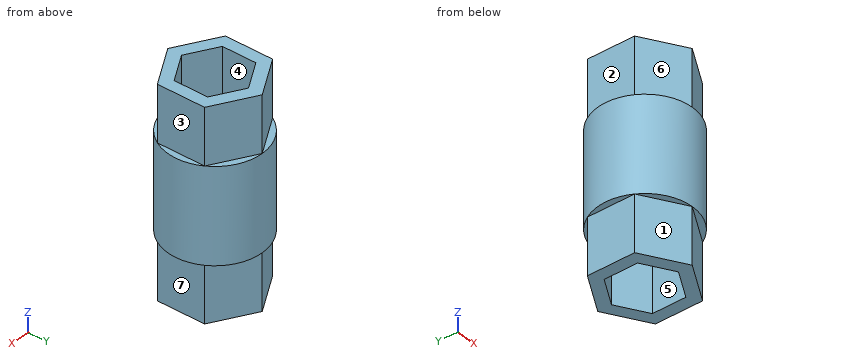
```python
from build123d import *

# Parameters (mm, degrees)
SKETCH1_R           = 11
SKETCH1_R_2         = 6.4
BOSS_EXTRUDE1_DEPTH = 11
BOSS_EXTRUDE2_DEPTH = 24
CUT_EXTRUDE3_DEPTH  = 49


with BuildPart() as part:
    # Sketch1 → Boss-Extrude1 (new body, symmetric)
    with BuildSketch(Plane.XY):
        Circle(SKETCH1_R)
        Circle(SKETCH1_R_2, mode=Mode.SUBTRACT)
    extrude(amount=BOSS_EXTRUDE1_DEPTH, both=True)

    # Sketch1_3 → Boss-Extrude2 (add, symmetric)
    with BuildSketch(Plane.XY):
        Polygon((0, -11), (9.526279442, -5.5), (9.526279442, 5.5), (0, 11), (-9.526279442, 5.5), (-9.526279442, -5.5), align=None)
    extrude(amount=BOSS_EXTRUDE2_DEPTH, both=True)

    # Sketch2 → Cut-Extrude3 (cut, through all)
    with BuildSketch(Plane.XY.offset(24)):
        Polygon((0, -7.8), (6.75499815, -3.9), (6.75499815, 3.9), (0, 7.8), (-6.75499815, 3.9), (-6.75499815, -3.9), align=None)
    extrude(amount=-CUT_EXTRUDE3_DEPTH, mode=Mode.SUBTRACT)


solid = part.part
```
Could you check a few things on this model? Use its own coordinates, in mm. Face numbers are marked on the shaded views. A direction names the side the tool comes from. Coordinates: 2 decimals unless noted, no trailing zeros. Order: outer loops, then holes, each group sorted by start corner. A loop starts at its lowest first (then second) coordinate and runs counter-clockwise, first axis right, second up. Notation, with made-up numbers: M -32,67 L 22,67 A30 ccw 22,104 Z; hole C 23.25,23 d6. An arc over 180 degrees is marked long. Use a Markdown table: item, result. Add a question column.
Q1. I'm going to push flat-ended pins straight in: pin 1 (9 mm diameter, centred on y = -2, z = 16.5, fed in from +X); pin 2 (8 mm diameter, centred on y = -4.5, z = 12.5, fed in from -X); pin 3 (1.6 mm diameter, centred on x = 10.5, y = 1, fed in from +Z). Where does each tip first touch, or does it pass through?
Q2. If I drill on L1, parallel to Y at x = 4, z = 7; L2, parallel to Y at x = 3.75, z = 14; L3, parallel to X at y = 2, z = 21.5 (3 decimals), over which ranges is the centre line in solid material (lowest first)?
Q3. I want a section at D-D on z = 17. List the corners of the cut face in (x, y) for me (3 decimals), then the cut area to 3 significant figures.
Q4. I want a section at C-C on x = 3.5. List the corners of the cut face in (y, z) for me, then the cut area to 3 significant figures.
Q5. We'd pull the mould along Y, two halves only. Please class the marked faces 5, 6 and 7: pulls with the +Y half, pulls with the -Y half, needs draft (parallel to the pull), parting line crosses it, or undercut.
Q6. I want a section at A-A on z = 2.5. List the corners of the cut face in (x, y) for me (3 decimals).
Q7. Which directions (+Z, -Z, +X, -X, +Y, -Y) give clear straight access to the entire face, cutting with the end or side of a thin tool? Please do the marked faces 1, 2, 3 and 4.
Q8. I want a section at B-B on y = 2.75. List the corners of the cut face in (x, z) for me (3 decimals).
Checked values:
| question | item | result |
|---|---|---|
| 1 | pin 1 | x = 9.53 |
| 1 | pin 2 | x = -10.97 |
| 1 | pin 3 | z = 11 |
| 2 | L1 | -10.25 to -5.49, 5.49 to 10.25 |
| 2 | L2 | -8.83 to -5.63, 5.63 to 8.83 |
| 2 | L3 | -9.526 to -6.755, 6.755 to 9.526 |
| 3 | outline | M -9.526,-5.5 L 0,-11 L 9.526,-5.5 L 9.526,5.5 L 0,11 L -9.526,5.5 Z; hole M -6.755,-3.9 L 0,-7.8 L 6.755,-3.9 L 6.755,3.9 L 0,7.8 L -6.755,3.9 Z |
| 3 | area | 156 mm² |
| 4 | outline | M -10.43,-11 L -8.98,-11 L -8.98,-24 L -5.78,-24 L -5.78,24 L -8.98,24 L -8.98,11 L -10.43,11 Z; M 5.78,-24 L 8.98,-24 L 8.98,-11 L 10.43,-11 L 10.43,11 L 8.98,11 L 8.98,24 L 5.78,24 Z |
| 4 | area | 371 mm² |
| 5 | face 5 | undercut |
| 5 | face 6 | pulls with the -Y half |
| 5 | face 7 | needs draft |
| 6 | outline | C 0,0 d22; hole M -6.755,-3.9 L 0,-7.8 L 6.755,-3.9 L 6.755,3.9 L 0,7.8 L -6.755,3.9 Z |
| 7 | face 1 | -Z, -X, -Y |
| 7 | face 2 | +Z, -X, +Y, -Y |
| 7 | face 3 | +Z, +X, +Y, -Y |
| 7 | face 4 | +Z, -Z |
| 8 | outline | M -10.651,-11 L -9.526,-11 L -9.526,-24 L -6.755,-24 L -6.755,24 L -9.526,24 L -9.526,11 L -10.651,11 Z; M 6.755,-24 L 9.526,-24 L 9.526,-11 L 10.651,-11 L 10.651,11 L 9.526,11 L 9.526,24 L 6.755,24 Z |
